Can you work these out from the model? Positions are in its coordinate system, mm. Give positions to 0.01 mm unless a question says otherwise; leave off trailing zeros. Write each loop counter-clockwise with the first axis right and the second up, starting at its lowest first coordinate (ties: lowest second). Pieces come first, ordered by that corner, then holes. Notation, with made-up numbers: (40, 59) -> (52, 59) arc R9 ccw to (52, 67) -> close; hole circle Ø6 at (21.25, -10). An arc over 180 degrees is marked (long way). One line per item, written item: value.
from build123d import *

# Parameters (mm, degrees)
BOSS_EXTRUDE1_DEPTH = 3


with BuildPart() as part:
    # Sketch1 → Boss-Extrude1 (new body)
    with BuildSketch(Plane(origin=(0, 0, 0), x_dir=(1, 0, 0), z_dir=(0, 1, 0))):
        with BuildLine():
            add(Edge.make_bspline(
                [(45.281536872, -37), (-12.284726177, -48.689174516), (-51.82483075, -92.30412262), (-105, -112.092029096)],
                knots=[0, 0, 0, 0, 1, 1, 1, 1], degree=3))
            Line((45.281536872, -37), (51.259707723, -37))
            Line((51.259707723, -37), (110, -112.392253356))
            Line((110, -112.392253356), (110, -17))
            Line((110, -17), (75, -17))
            Line((75, -17), (75, 37))
            Line((75, 37), (-75, 37))
            Line((-75, 37), (-75, -17))
            Line((-75, -17), (-105, -17))
            Line((-105, -17), (-105, -112.092029096))
        make_face()
    extrude(amount=BOSS_EXTRUDE1_DEPTH)


solid = part.part
1) If we section it at B-B (x = 84): Write out the boundary of the cut face in (y, z).
Answer list:
outline: (0, 17) -> (3, 17) -> (3, 79.02) -> (0, 79.02) -> close
2) We'd pull the mould along X, two halves only. Please class faces 1 (the face through (80.22, 1.48, 74.17)), 2 (the face through (4, 3, 20)): released by +X, released by -X, zero draft, split by the parting line, or undercut.
Answer list:
face 1: undercut
face 2: zero draft
3) I need wall thicknesses on L1, parallel to X at y = 1.15, z = 85; L2, parallel to X at y = 2.85, z = 8; L3, parallel to X at y = 1.35, z = 49. Which ranges of each line are inside material? Lowest first, please.
Answer list:
L1: x = -105 to -52.9, 88.66 to 110
L2: x = -75 to 75
L3: x = -105 to 9.03, 60.61 to 110
4) Will these pins go through, and if not, where does the flat tip stop? pin 1 (1.5 mm diameter, centred on x = 95.5, y = 1.5, fed in from -Z); pin 2 (1.5 mm diameter, centred on y = 2, z = -18.5, fed in from -X); pin 3 (1.5 mm diameter, centred on x = -66.5, y = 0.5, fed in from +Z).
Answer list:
pin 1: stops at z = 17
pin 2: stops at x = -75
pin 3: stops at z = 93.7
5) If we section it at A-A (z = -8): Write out the boundary of the cut face in (x, y), and give its area (3 significant figures).
Answer list:
outline: (-75, 0) -> (75, 0) -> (75, 3) -> (-75, 3) -> close
area: 450 mm^2
